```python
from build123d import *

# Parameters (mm, degrees)
SKETCH1_W            = 16.2
SKETCH1_H            = 16
SKETCH1_R            = 2
BOSS_EXTRUDE3_DEPTH  = 2
SKETCH1_3_W          = 3
SKETCH1_3_H          = 2.5
BOSS_EXTRUDE4_DEPTH  = 25.5
SKETCH1_4_W          = 2
SKETCH1_4_H          = 2
BOSS_EXTRUDE5_DEPTH  = 1.5
SKETCH1_8_W          = 13.2
SKETCH1_8_H          = 2.5
BOSS_EXTRUDE6_DEPTH  = 2
SKETCH1_9_W          = 13.2
SKETCH1_9_H          = 4
SKETCH1_9_W_2        = 3
BOSS_EXTRUDE7_DEPTH  = 2
SKETCH1_11_W         = 3
SKETCH1_11_H         = 2.5
SKETCH1_11_W_2       = 13.2
BOSS_EXTRUDE9_DEPTH  = 10.5
SKETCH1_12_W         = 13.2
SKETCH1_12_H         = 2.5
BOSS_EXTRUDE10_DEPTH = 25.5


with BuildPart() as part:
    # Sketch1 → Boss-Extrude3 (new body)
    with BuildSketch(Plane.XY):
        with Locations((0, -4.5)):
            Rectangle(SKETCH1_W, SKETCH1_H)
        with Locations((0, -7.5)):
            Circle(SKETCH1_R, mode=Mode.SUBTRACT)
    extrude(amount=BOSS_EXTRUDE3_DEPTH)

    # Sketch1<4> → Boss-Extrude5 (add)
    with BuildSketch(Plane.XY):
        with Locations((0, -1.5)):
            Rectangle(SKETCH1_4_W, SKETCH1_4_H)
    extrude(amount=-BOSS_EXTRUDE5_DEPTH)



with BuildPart() as body_2:
    # Sketch1<3> → Boss-Extrude4 (new body)
    with BuildSketch(Plane.XY):
        with Locations((-6.6, 8.75)):
            Rectangle(SKETCH1_3_W, SKETCH1_3_H)
    extrude(amount=BOSS_EXTRUDE4_DEPTH)


with BuildPart() as body_3:
    # Sketch1<8> → Boss-Extrude6 (new body)
    with BuildSketch(Plane.XY):
        with Locations((1.5, 8.75)):
            Rectangle(SKETCH1_8_W, SKETCH1_8_H)
    extrude(amount=BOSS_EXTRUDE6_DEPTH)


with BuildPart() as part_1:
    add(part.part)

    add(body_2.part)  # Boss-Extrude7 merges body 2

    add(body_3.part)  # Boss-Extrude7 merges body 3
    # Sketch1<9> → Boss-Extrude7 (add)
    with BuildSketch(Plane.XY):
        with Locations((1.5, 5.5)):
            Rectangle(SKETCH1_9_W, SKETCH1_9_H)
        with Locations((-6.6, 5.5)):
            Rectangle(SKETCH1_9_W_2, SKETCH1_9_H)
    extrude(amount=BOSS_EXTRUDE7_DEPTH)

    # Sketch1<11> → Boss-Extrude9 (add)
    with BuildSketch(Plane.XY):
        with Locations((-6.6, 11.25)):
            Rectangle(SKETCH1_11_W, SKETCH1_11_H)
        with Locations((1.5, 11.25)):
            Rectangle(SKETCH1_11_W_2, SKETCH1_11_H)
    extrude(amount=BOSS_EXTRUDE9_DEPTH)

    # Sketch1<12> → Boss-Extrude10 (add)
    with BuildSketch(Plane.XY):
        with Locations((1.5, 8.75)):
            Rectangle(SKETCH1_12_W, SKETCH1_12_H)
    extrude(amount=BOSS_EXTRUDE10_DEPTH)


solid = part_1.part
```
Verification items for the finished model (mm, model axes). A direction names the side the tool comes from. Give positions to 0.01 mm unless a question says otherwise; leave off trailing zeros. Order: outer loops, then holes, each group sorted by start corner. A loop starts at its lowest first (then second) coordinate and runs counter-clockwise, first axis right, second up. Notation, with made-up numbers: (-16.75, 77) - (0.25, 77) arc R21 cw to (0.25, 108) - close; hole circle Ø10 at (6, 15). An arc over 180 degrees is marked (long way). Answer as CSV lines item,"result". Start each with the question number.
Item 1: Material ranges on L1, parallel to Y at x = 0, z = 0.55; L2, parallel to Z at x = -1.75, y = -0.5; L3, parallel to Y at x = -5.75, z = 12.25, recorded low to high.
Item 2: Section check B-B, the plane y = -7.5. Record the boundary of the cut face in (x, z).
Item 3: Section check C-C, the plane x = -5.75. Record the boundary of the cut face in (y, z), plus the area to 3 significant figures.
Item 4: Mould release check, pull along X, two halves, no side actions. Record for faces 5 (the face through (0, -2, 2)), 6 (the face through (8.1, 8, 6)), 7 (the face through (-0.26, -5.517, 0.986)): released by +X, released by -X, zero draft, split by the parting line, or undercut.
Item 5: Gauge pin test, flat ends, axial feed: pin 1 (5 mm diameter, centred on x = -0.5, y = -9, fed in from -Z); pin 2 (8 mm diameter, centred on x = -0.5, z = 14.5, fed in from -Y); pin 3 (0.8 mm diameter, centred on x = 3, y = 11, fed in from +Z); pin 4 (8 mm diameter, centred on y = 0.5, z = 11, fed in from -X). Record the tip position at first contact, or that the pin passes through.
Item 6: Access from +Z, -Z, +X, -X, +Y, -Y to the whole of each face (thin tool, end or side, straight path). Record for faces 1 (the face through (1, -2, -1)), 2 (the face through (0, 10, 18)), 3 (the face through (0, 7.5, 14)), 4 (the face through (-1, -2, -1)).
Item 7: Section check D-D, the plane z = 12.75. Record the boundary of the cut face in (x, y), plus the area to 3 significant figures.
Item 8: Section check A-A, the plane x = 0. Record the boundary of the cut face in (y, z).
Filled in:
1,L1,"-12.5 to -9.5, -5.5 to 12.5"
1,L2,"0 to 2"
1,L3,"7.5 to 10"
2,outline,"(-8.1, 0) - (-2, 0) - (-2, 2) - (-8.1, 2) - close; (2, 0) - (8.1, 0) - (8.1, 2) - (2, 2) - close"
3,outline,"(-12.5, 0) - (12.5, 0) - (12.5, 10.5) - (10, 10.5) - (10, 25.5) - (7.5, 25.5) - (7.5, 2) - (-12.5, 2) - close"
3,area,"130 mm^2"
4,face 5,"zero draft"
4,face 6,"released by +X"
4,face 7,"undercut"
5,pin 1,"z = 0"
5,pin 2,"y = 7.5"
5,pin 3,"z = 10.5"
5,pin 4,"through"
6,face 1,"-Z, +X, +Y, -Y"
6,face 2,"+Z, +X, -X, +Y"
6,face 3,"+Z, +X, -X, -Y"
6,face 4,"-Z, -X, +Y, -Y"
7,outline,"(-8.1, 7.5) - (8.1, 7.5) - (8.1, 10) - (-8.1, 10) - close"
7,area,"40.5 mm^2"
8,outline,"(-12.5, 0) - (-9.5, 0) - (-9.5, 2) - (-12.5, 2) - close; (-5.5, 0) - (-2.5, 0) - (-2.5, -1.5) - (-0.5, -1.5) - (-0.5, 0) - (12.5, 0) - (12.5, 10.5) - (10, 10.5) - (10, 25.5) - (7.5, 25.5) - (7.5, 2) - (-5.5, 2) - close"
